```python
from build123d import *

# Parameters (mm, degrees)
F1_DEPTH = 10
F2_DEPTH = 6.3
F3_R     = 1.6
F4_DEPTH = 25
F5_DEPTH = 1
F6_DEPTH = 0.25


with BuildPart() as f1:
    # F0 (on Top) → F1 (new body)
    with BuildSketch(Plane.XY):
        with BuildLine():
            ThreePointArc((-8.125, 0), (0, 8.125), (8.125, 0))
            Line((8.125, 0), (15, 0))
            Line((15, 0), (15, 10))
            Line((15, 10), (-27, 10))
            Line((-27, 10), (-27, 0))
            Line((-27, 0), (-8.125, 0))
        make_face()
    extrude(amount=-F1_DEPTH)

    # F0 (on Top) → F2 (join)
    with BuildSketch(Plane.XY):
        with BuildLine():
            ThreePointArc((-6.15, 0), (0, 6.15), (6.15, 0))
            Line((6.15, 0), (8.125, 0))
            ThreePointArc((8.125, 0), (0, 8.125), (-8.125, 0))
            Line((-8.125, 0), (-6.15, 0))
        make_face()
    extrude(amount=-F2_DEPTH)

    # F3 (on face) → F4 (cut)
    with BuildSketch(Plane(origin=(0, 10, 0), x_dir=(-1, 0, 0), z_dir=(0, 1, 0))):
        with Locations((-9.5, -5.5)):
            Circle(F3_R)
        with BuildLine():
            ThreePointArc((23.1, -5.5), (21.5, -3.9), (19.9, -5.5))
            ThreePointArc((19.9, -5.5), (21.5, -7.1), (23.1, -5.5))
        make_face()
    extrude(amount=-F4_DEPTH, mode=Mode.SUBTRACT)

    # F0 (on Top) → F5 (cut)
    with BuildSketch(Plane.XY):
        with BuildLine():
            ThreePointArc((-8.125, 0), (0, 8.125), (8.125, 0))
            Line((8.125, 0), (15, 0))
            Line((15, 0), (15, 10))
            Line((15, 10), (-27, 10))
            Line((-27, 10), (-27, 0))
            Line((-27, 0), (-8.125, 0))
        make_face()
        with BuildLine():
            ThreePointArc((-6.15, 0), (0, 6.15), (6.15, 0))
            Line((6.15, 0), (8.125, 0))
            ThreePointArc((8.125, 0), (0, 8.125), (-8.125, 0))
            Line((-8.125, 0), (-6.15, 0))
        make_face()
    extrude(amount=-F5_DEPTH, mode=Mode.SUBTRACT)

    # F6 (cut): a face of the model
    f6_faces = [f1.faces().sort_by_distance(p)[0] for p in [
        (-7.1375, 0.1815853566, -6.3),
    ]]
    extrude(f6_faces, amount=-F6_DEPTH, mode=Mode.SUBTRACT)


solid = f1.part
```
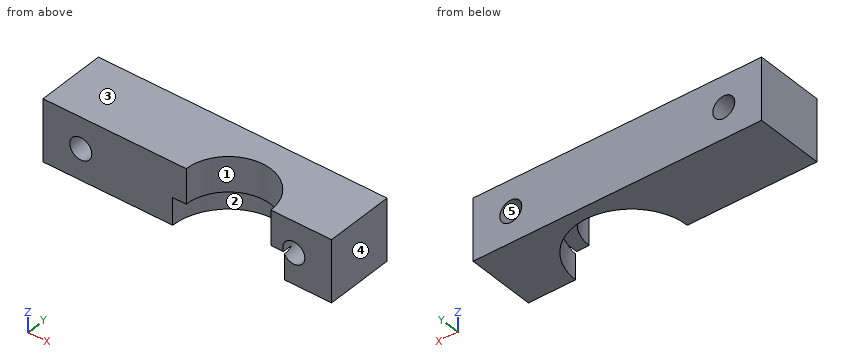
Input: part model. Units: mm. Frame: model coordinates. Face numbers are marked on the shaded views. A direction names the side the tool comes from. Coordinates: 2 decimals unless noted, no trailing zeros. Loops run counter-clockwise (first coordinate to the right, second up) from the corner with the lowest first, then second, coordinate; pieces in that order, holes last. Notation, with made-up numbers: (1, 83.5) - (46, 83.5) arc R12 ccw to (46, 101.5) - close; hole circle Ø6 at (66, -20.75). An arc over 180 degrees is marked (long way). Answer in a Markdown table with one row per item.
(1) Pin query (flat end, axial travel): P1, Ø3, axis at x = 1, z = -9, coming from the -Y side; P2, Ø3, axis at x = -21.5, z = -5.5, coming from the -Y side. Return the tip coordinate at first contact, or that it passes through.
Model answer:
| item | result |
|---|---|
| P1 | stops at y = 7.73 |
| P2 | passes through |
(2) Mould query, pull axis X, two halves, no side actions, for the marked faces 3, 4 and 5. Classes: pulls with the +X half, pulls with the -X half, needs draft (parallel to the pull), parting line crosses it, or undercut.
Model answer:
| item | result |
|---|---|
| face 3 | needs draft |
| face 4 | pulls with the +X half |
| face 5 | undercut |
(3) Cut plane D-D on z = -2.5. Output: boundary loops of the cut face in (x, y).
Model answer:
| item | result |
|---|---|
| outline | (-27, 0) - (-6.15, 0) arc R6.15 cw to (6.15, 0) - (15, 0) - (15, 10) - (-27, 10) - close |
(4) Cut plane A-A on z = -5.5. Output: boundary loops of the cut face in (x, y).
Model answer:
| item | result |
|---|---|
| outline | (-27, 0) - (-23.1, 0) - (-23.1, 10) - (-27, 10) - close; (-19.9, 0) - (-6.15, 0) arc R6.15 cw to (6.15, 0) - (7.9, 0) - (7.9, 10) - (-19.9, 10) - close; (11.1, 0) - (15, 0) - (15, 10) - (11.1, 10) - close |
(5) Cut plane B-B on x = 9.5. Output: boundary loops of the cut face in (y, z).
Model answer:
| item | result |
|---|---|
| outline | (0, -10) - (10, -10) - (10, -7.1) - (0, -7.1) - close; (0, -3.9) - (10, -3.9) - (10, -1) - (0, -1) - close |
(6) Set-up query: the marked faces 1 and 2. Return all of +Z, -Z, +X, -X, +Y, -Y with unobstructed straight access to the full face (end or side cutting, diameter ignored); none if empty.
Model answer:
| item | result |
|---|---|
| face 1 | +Z, -Z, -Y |
| face 2 | -Z, -Y |
(7) Material intervals for L1, parallel to Z at x = 9.5, y = 4.75; L2, parallel to X at y = 4, z = -5.5; L3, parallel to X at y = 4.75, z = -5.5, sorted ascending. Write a range as from..to.
Model answer:
| item | result |
|---|---|
| L1 | z = -10..-7.1, -3.9..-1 |
| L2 | x = -27..-23.1, -19.9..-4.67, 4.67..7.9, 11.1..15 |
| L3 | x = -27..-23.1, -19.9..-3.91, 3.91..7.9, 11.1..15 |
(8) Cut plane C-C on y = 3.5. Output: boundary loops of the cut face in (x, z).
Model answer:
| item | result |
|---|---|
| outline | (-27, -10) - (-7.33, -10) - (-7.33, -6.05) - (-5.06, -6.05) - (-5.06, -1) - (-27, -1) - close; (5.06, -6.05) - (7.33, -6.05) - (7.33, -10) - (15, -10) - (15, -1) - (5.06, -1) - close; hole circle Ø3.2 at (-21.5, -5.5); hole circle Ø3.2 at (9.5, -5.5) |
